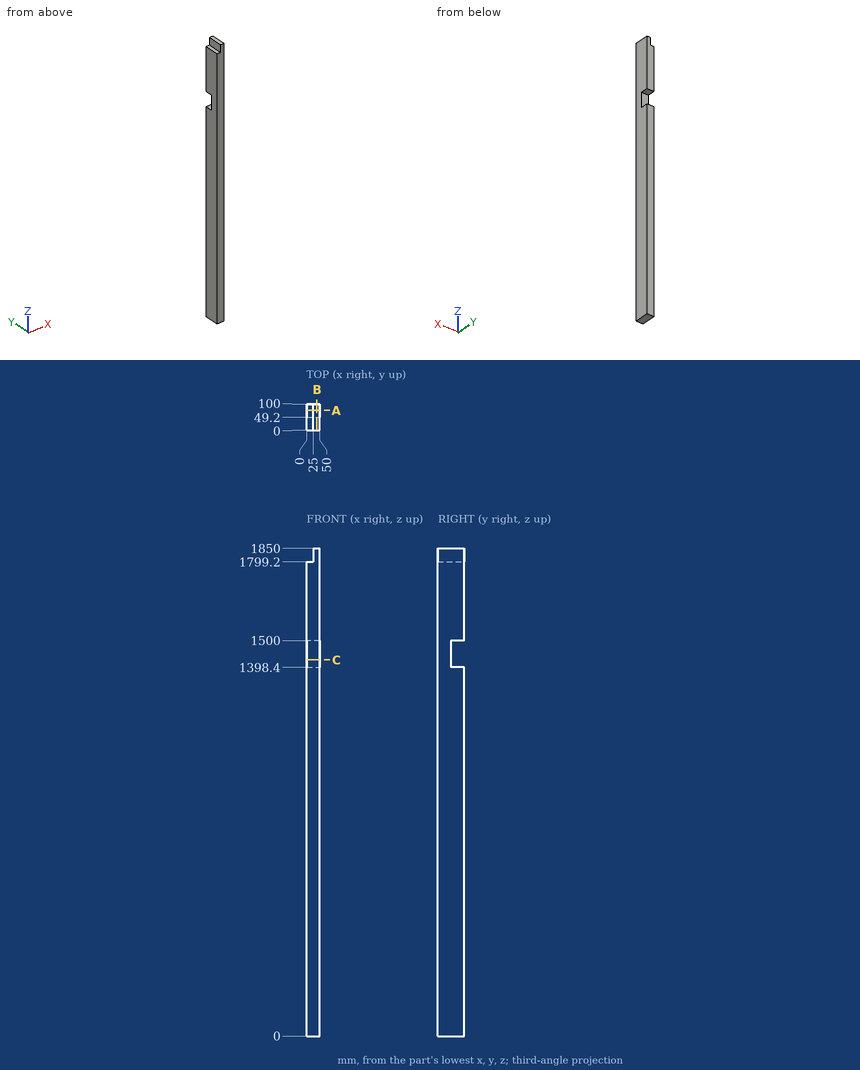
Study the drawing (mm; zero at the part's minimum x, y, z) and answer. Give positions to 0.01 mm unless a question says otherwise; leave off trailing zeros. Order: outer loops, then holes, each group sorted by start corner. A loop starts at its lowest first (then second) coordinate and runs counter-clockwise, first axis right, second up. Notation, with made-up numbers: (85.25, 67.5) - (117.25, 67.5) arc R25 ccw to (117.25, 87.5) - close; hole circle Ø2 at (50, 73.5). An arc over 180 degrees is marked (long way). Use one line per item in the form item = value. Start each with the question number.
(1) Consider line 1 (Z direction, x = 11, y = 66.5); line 2 (Z direction, x = 45, y = 79.5); line 3 (Y direction, x = 31, z = 1462). Determine where each line is inside the solid, lowest interval first. Write a range as from..to.
(2) A cutting plane is placed at A-A, the plane y = 75.5. Write down the section's boundary in (x, z).
(3) A cutting plane is placed at B-B, the plane x = 38. Write down the section's boundary in (y, z).
(4) Flat-ended cylindrical pins translate along their axes: pin 1 Ø1 at (x, z) = (31.5, 1474.5) entering from -Y; pin 2 Ø6 at (x, y) = (10, 83.5) entering from +Z; pin 3 Ø25 at (x, z) = (13, 1456.5) entering from +Y. Find the tip coordinate at first contact, or state that the pin passes through.
(5) A cutting plane is placed at C-C, the plane z = 1427. Write down the section's boundary in (x, y).
Ans:
q1.line_1 = 0..1398.4, 1500..1799.2
q1.line_2 = 0..1398.4, 1500..1850
q1.line_3 = 0..49.2
q2.outline = (0, 0) - (50, 0) - (50, 1398.4) - (0, 1398.4) - close; (0, 1500) - (50, 1500) - (50, 1850) - (25, 1850) - (25, 1799.2) - (0, 1799.2) - close
q3.outline = (0, 0) - (100, 0) - (100, 1398.4) - (49.2, 1398.4) - (49.2, 1500) - (100, 1500) - (100, 1850) - (0, 1850) - close
q4.pin_1 = 0
q4.pin_2 = 1799.2
q4.pin_3 = 49.2
q5.outline = (0, 0) - (50, 0) - (50, 49.2) - (0, 49.2) - close
